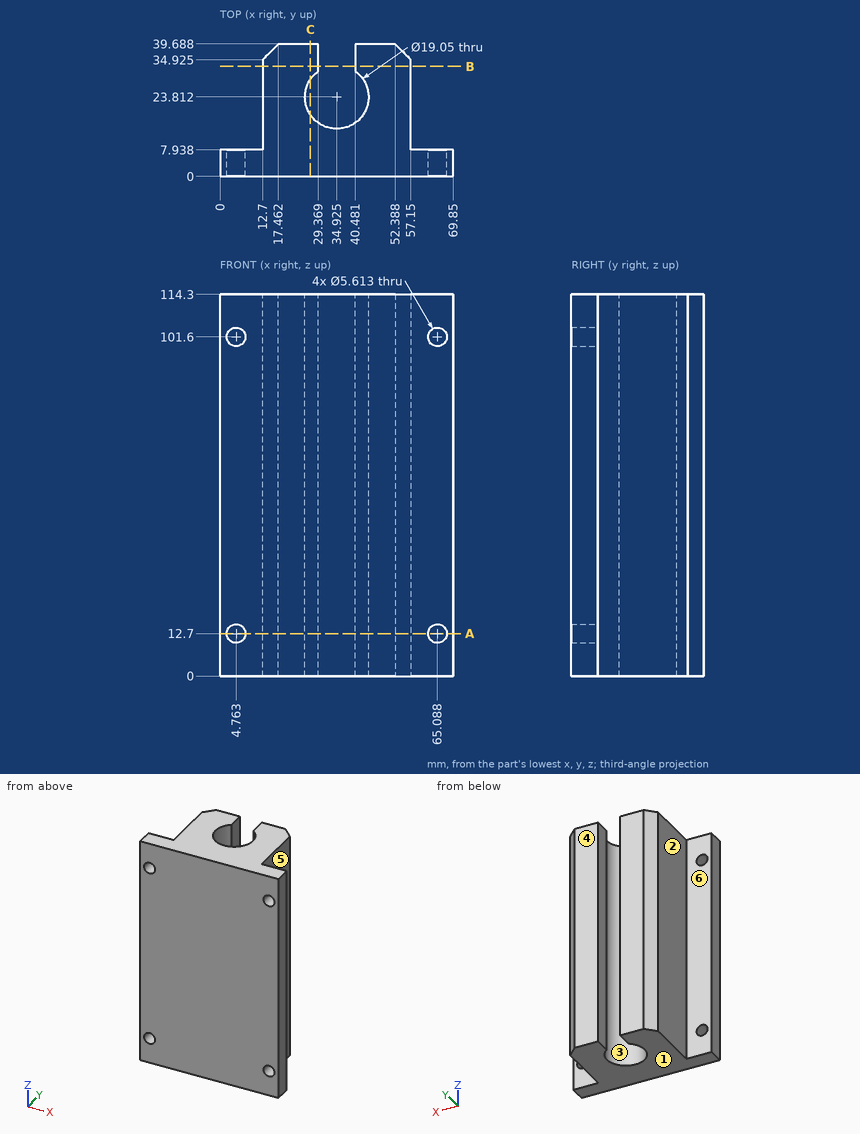
Here's the drawing with two shaded views (mm, measured from the low corner). I have some questions. A direction names the side the tool comes from. Coordinates: 2 decimals unless noted, no trailing zeros. Write each loop counter-clockwise with the first axis right and the second up, starting at its lowest first coordinate (ties: lowest second). Pieces come first, ordered by that corner, then holes. Notation, with made-up numbers: (29, 31) - (84, 31) arc R23 ccw to (84, 59) - close; hole circle Ø11 at (35, 87). An arc over 180 degrees is marked (long way). Return JSON: item names as keys, results as strings.
Q1. If we section it at B-B (y = 33): Please give me the cut outline in (x, z), then the cut area to 3 significant figures.
Computed values:
{"outline": "(12.7, 0) - (29.37, 0) - (29.37, 114.3) - (12.7, 114.3) - close; (40.48, 0) - (57.15, 0) - (57.15, 114.3) - (40.48, 114.3) - close", "area": "3,810 mm2"}
Q2. If we section it at C-C (x = 27): Please give me the cut outline in (y, z), then the cut area to 3 significant figures.
Computed values:
{"outline": "(0, 0) - (18.53, 0) - (18.53, 114.3) - (0, 114.3) - close; (29.1, 0) - (39.69, 0) - (39.69, 114.3) - (29.1, 114.3) - close", "area": "3,330 mm2"}
Q3. Please list where these lines run through material, in increasing order: L1, parallel to X at y = 33.5, z = 81.5; L2, parallel to Y at x = 61.5, z = 30; L3, parallel to Z at x = 7, y = 3.5 (1 decimal). Write a range as from..to.
Computed values:
{"L1": "x = 12.7..29.37, 40.48..57.15", "L2": "y = 0..7.94", "L3": "z = 0..11, 14.4..99.9, 103.3..114.3"}
Q4. If we section it at A-A (z = 12.7): Count the separate pieces of the cut face and the enclosed holes in it, then the cut area to 3 significant figures.
Computed values:
{"separate pieces": "3", "enclosed holes": "0", "area": "1,490 mm2"}
Q5. Thinking about a two-plate mould opening in X: for the marked faces 1, 2 and 3, which applies, +X half, -X half, draft (parallel to the pull), parting line (faces both ways), or undercut?
Computed values:
{"face 1": "draft", "face 2": "-X half", "face 3": "undercut"}
Q6. On a 3-axis mill with a long thin cutter (end or side, diameter ignored), from which of +Z, -Z, +X, -X, +Y, -Y can I reach the whole of each face in a straight line? I mean the marked faces 4, 5 and 6. Say none if no direction works.
Computed values:
{"face 4": "+Z, -Z, +X, -X, +Y", "face 5": "+Z, -Z, +X, +Y", "face 6": "+Z, -Z, -X, +Y"}
Q7. I'm going to push flat-ended pins straight in: pin 1 Ø10 at (y, z) = (21, 95.5) entering from +X; pin 2 Ø1 at (x, z) = (55.5, 43.5) entering from +Y (1 decimal); pin 3 Ø5 at (x, y) = (41, 22.5) entering from +Z; pin 4 Ø4 at (x, z) = (65.5, 79.5) entering from +Y. Where does each tip first touch, or does it pass through?
Computed values:
{"pin 1": "stops at x = 57.15", "pin 2": "stops at y = 37.1", "pin 3": "passes through", "pin 4": "stops at y = 7.94"}
